Can you work these out from the model? Positions are in its coordinate system, mm. Coordinates: 2 decimals unless noted, no trailing zeros. Write each loop counter-clockwise with the first axis right and the second up, starting at its lowest first coordinate (ties: lowest second). Pieces come first, ordered by that corner, then holes. Notation, with made-up numbers: M 59,7 L 103,7 A10 ccw 103,17 Z; hole C 75,66.5 d1. An arc over 180 degrees is marked long. Answer as a JSON object with one key per item and string values. Group by question number.
from build123d import *

# Parameters (mm, degrees)
BOSS_EXTRUDE1_DEPTH     = 10
CUT_EXTRUDE4_DEPTH      = 11
CUT_EXTRUDE4_DEPTH_BACK = 1


with BuildPart() as part:
    # Sketch1 → Boss-Extrude1 (new body)
    with BuildSketch(Plane(origin=(0, 0, 0), x_dir=(1, 0, 0), z_dir=(0, 1, 0))):
        with BuildLine():
            Line((0, -5), (0, -37.596875763))
            ThreePointArc((0, -37.596875763), (0.493483818, -39.762819415), (1.876524762, -41.50121981))
            Line((1.876524762, -41.50121981), (23.630430059, -58.904344047))
            ThreePointArc((23.630430059, -58.904344047), (25.09887059, -59.718141596), (26.753905297, -60))
            Line((26.753905297, -60), (273.246094703, -60))
            ThreePointArc((273.246094703, -60), (274.90112941, -59.718141596), (276.369569941, -58.904344047))
            Line((276.369569941, -58.904344047), (298.123475238, -41.50121981))
            ThreePointArc((298.123475238, -41.50121981), (299.506516182, -39.762819415), (300, -37.596875763))
            Line((300, -37.596875763), (300, -5))
            ThreePointArc((300, -5), (298.535533906, -1.464466094), (295, 0))
            Line((295, 0), (5, 0))
            ThreePointArc((5, 0), (1.464466094, -1.464466094), (0, -5))
        make_face()
    extrude(amount=BOSS_EXTRUDE1_DEPTH)

    # Sketch2 → Cut-Extrude4 (cut, two sides)
    with BuildSketch(Plane(origin=(0, 0, 0), x_dir=(1, 0, 0), z_dir=(0, 1, 0))) as cut_extrude4_sk:
        with BuildLine():
            Line((25, -44), (275, -44))
            ThreePointArc((275, -44), (278, -47), (275, -50))
            Line((275, -50), (25, -50))
            ThreePointArc((25, -50), (22, -47), (25, -44))
        make_face()
    extrude(amount=CUT_EXTRUDE4_DEPTH, mode=Mode.SUBTRACT)
    extrude(cut_extrude4_sk.sketch, amount=-CUT_EXTRUDE4_DEPTH_BACK, mode=Mode.SUBTRACT)


solid = part.part
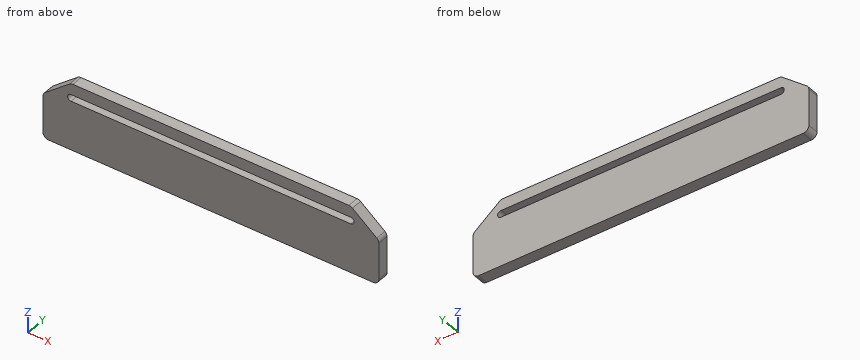
Q1. Please list where these lines run through material, in increasing order: L1, parallel to Z at x = 33, y = 7.25; L2, parallel to X at y = 3.5, z = 45.5 (3 decimals); L3, parallel to X at y = 6.5, z = 44.5 (3 decimals).
Q2. If we section it at B-B on x = 148: List the corners of the cut face in (y, z) for me.
Q3. If we section it at A-A on y = 7.75: List the corners of the cut face in (x, z) for me.
Q4. If we section it at C-C on z = 47: List the corners of the cut face in (x, y) for me, and give its area (3 significant figures).
Reply:
{
 "1": {"L1": "0 to 44, 50 to 60", "L2": "6.875 to 22.402, 277.598 to 293.125", "L3": "5.625 to 23.342, 276.658 to 294.375"},
 "2": {"outline": "M 0,0 L 10,0 L 10,44 L 0,44 Z; M 0,50 L 10,50 L 10,60 L 0,60 Z"},
 "3": {"outline": "M 0,5 A5 ccw 5,0 L 295,0 A5 ccw 300,5 L 300,37.6 A5 ccw 298.12,41.5 L 276.37,58.9 A5 ccw 273.25,60 L 26.75,60 A5 ccw 23.63,58.9 L 1.88,41.5 A5 ccw 0,37.6 Z; hole M 25,44 L 275,44 A3 ccw 275,50 L 25,50 A3 ccw Z"},
 "4": {"outline": "M 8.75,0 L 22,0 L 22,10 L 8.75,10 Z; M 278,0 L 291.25,0 L 291.25,10 L 278,10 Z", "area": "265 mm^2"}
}
